Part model, mm, in its own coordinate system. A direction names the side the tool comes from. Round coordinates to 2 decimals unless told otherwise and drop trailing zeros. Write each loop counter-clockwise with the first axis right and the second up, starting at its lowest first coordinate (ties: lowest second). Pieces come first, ordered by that corner, then holes. Notation, with made-up numbers: M 6,-9.5 L 28,-9.5 A34 ccw 28,23.5 Z; hole C 73.5,-37.5 d11. An arc over 180 degrees is marked long. Use a Markdown table: item, result. Add a question column.
1) Slice it at C-C on z = 12. Write the cut outline in (x, y), plus the area to 3 significant figures.
2) Two-plate mould, pull along Y, no slides. Class faces 5 (the face through (-0.5, 2, 13)), 6 (the face through (0, -4, 0)), 7 (the face through (-0.9, 0, 0.2)): released by +Y, released by -Y, zero draft, split by the parting line, or undercut.
3) Slice it at D-D on x = -3. Write the cut outline in (y, z).
4) Which spindle directions (+Z, -Z, +X, -X, +Y, -Y) get a long thin tool onto all of the face, cutting with end or side? Do faces 1 (the face through (0.5, -2, 13)), 2 (the face through (2, 0, 10)), 3 (the face through (2, 0.5, -13)), 4 (the face through (-0.5, 2, -13)). Say none if no direction does.
5) Drop a flat-ended pin along its axis: P1, Ø0.8, axis at x = 0, y = 2, coming from the -Z side. Give the stop position or say it passes through.
6) Wall check: probe 1 along Y at (x, z) = (0, -7.5); probe 2 along X at (y, z) = (2, 11.75). Give the ranges that are in metal, low to high.
7) Slice it at A-A on y = 0. Write the cut outline in (x, z), plus the area to 3 significant figures.
```python
from build123d import *

# Parameters (mm, degrees)
F0_W          = 8
F0_H          = 8
F1_DEPTH      = 15
F1_DEPTH_BACK = 15
F2_R          = 0.9
F3_DEPTH      = 36.9
F4_W          = 4.5
F4_H          = 1
F4_W_2        = 1
F4_H_2        = 4.5
F5_DEPTH      = 5


# Not quite as in the source:
# - a pattern or mirror of a feature is missing from the dataset's text; its kind, count and spacing are read off the source's solid


with BuildPart() as f1:
    # F0 (on Top) → F1 (new body, two sides)
    with BuildSketch(Plane.XY) as f1_sk:
        Rectangle(F0_W, F0_H)
    extrude(amount=F1_DEPTH)
    extrude(f1_sk.sketch, amount=-F1_DEPTH_BACK)

    # F2 (on face) → F3 (cut)
    with BuildSketch(Plane.XY.offset(15)):
        Circle(F2_R)
    extrude(amount=-F3_DEPTH, mode=Mode.SUBTRACT)

    # F4 (on face) → F5 (cut)
    with BuildSketch(Plane.XY.offset(15)):
        with Locations((-2.75, 0)):
            Rectangle(F4_W, F4_H)
        Rectangle(F4_W_2, F4_H)
        with Locations((0, -2.75)):
            Rectangle(F4_W_2, F4_H_2)
        with Locations((2.75, 0)):
            Rectangle(F4_W, F4_H)
        with Locations((0, 2.75)):
            Rectangle(F4_W_2, F4_H_2)
    f5 = extrude(amount=-F5_DEPTH, mode=Mode.SUBTRACT)

    # F5_copies: F5 across plane
    add(f5.mirror(Plane(origin=(0, 0, 0), x_dir=(-1, 0, 0), z_dir=(0, 0, -1))), mode=Mode.SUBTRACT)


solid = f1.part
```
Entries:
| question | item | result |
|---|---|---|
| 1 | outline | M -4,-4 L -0.5,-4 L -0.5,-0.75 A0.9 cw -0.75,-0.5 L -4,-0.5 Z; M -4,0.5 L -0.75,0.5 A0.9 cw -0.5,0.75 L -0.5,4 L -4,4 Z; M 0.5,-4 L 4,-4 L 4,-0.5 L 0.75,-0.5 A0.9 cw 0.5,-0.75 Z; M 0.5,0.75 A0.9 cw 0.75,0.5 L 4,0.5 L 4,4 L 0.5,4 Z |
| 1 | area | 48.9 mm^2 |
| 2 | face 5 | zero draft |
| 2 | face 6 | released by -Y |
| 2 | face 7 | undercut |
| 3 | outline | M -4,-15 L -0.5,-15 L -0.5,-10 L 0.5,-10 L 0.5,-15 L 4,-15 L 4,15 L 0.5,15 L 0.5,10 L -0.5,10 L -0.5,15 L -4,15 Z |
| 4 | face 1 | +Z, +Y, -Y |
| 4 | face 2 | +Z, +X, -X |
| 4 | face 3 | -Z, +X, -X |
| 4 | face 4 | -Z, +Y, -Y |
| 5 | P1 | stops at z = -10 |
| 6 | probe 1 | y = -4 to -0.9, 0.9 to 4 |
| 6 | probe 2 | x = -4 to -0.5, 0.5 to 4 |
| 7 | outline | M -4,-10 L -0.9,-10 L -0.9,10 L -4,10 Z; M 0.9,-10 L 4,-10 L 4,10 L 0.9,10 Z |
| 7 | area | 124 mm^2 |
